```python
from build123d import *

# Parameters (mm, degrees)
BOSS_EXTRUDE1_DEPTH        = 5
BOSS_EXTRUDE1_DEPTH_BACK   = 5
BOSS_EXTRUDE1_2_DEPTH      = 5
BOSS_EXTRUDE1_2_DEPTH_BACK = 5
BOSS_EXTRUDE1_3_DEPTH      = 5
BOSS_EXTRUDE1_3_DEPTH_BACK = 5
BOSS_EXTRUDE2_DEPTH        = 10
BOSS_EXTRUDE2_DEPTH_BACK   = 10
SKETCH1_6_R                = 40
SKETCH1_6_R_2              = 25


with BuildPart() as part:
    # Sketch1 → Boss-Extrude1 (new, two sides: drawn at the far end of the back side and taken through both)
    with BuildSketch(Plane.XY.offset(-BOSS_EXTRUDE1_DEPTH_BACK)):
        with BuildLine():
            Line((10, 47.870166538), (10, -47.870166538))
            ThreePointArc((10, -47.870166538), (0, -46.6), (-10, -47.870166538))
            Line((-10, -47.870166538), (-10, 47.870166538))
            ThreePointArc((-10, 47.870166538), (0, 46.6), (10, 47.870166538))
        make_face()
    extrude(amount=BOSS_EXTRUDE1_DEPTH + BOSS_EXTRUDE1_DEPTH_BACK)



with BuildPart() as body_2:
    # Sketch1 → Boss-Extrude1 2 (new, two sides: drawn at the far end of the back side and taken through both)
    with BuildSketch(Plane.XY.offset(-BOSS_EXTRUDE1_2_DEPTH_BACK)):
        with BuildLine():
            Line((-122.049730922, 28.614375032), (-38.604515092, 76.126633087))
            ThreePointArc((-38.604515092, 76.126633087), (-34.719424314, 66.736425918), (-28.593413405, 58.628287327))
            Line((-28.593413405, 58.628287327), (-111.528626884, 10.952326263))
            ThreePointArc((-111.528626884, 10.952326263), (-115.635110511, 20.470817531), (-122.049730922, 28.614375032))
        make_face()
    extrude(amount=BOSS_EXTRUDE1_2_DEPTH + BOSS_EXTRUDE1_2_DEPTH_BACK)


with BuildPart() as body_3:
    # Sketch1 → Boss-Extrude1 3 (new, two sides: drawn at the far end of the back side and taken through both)
    with BuildSketch(Plane.XY.offset(-BOSS_EXTRUDE1_3_DEPTH_BACK)):
        with BuildLine():
            Line((-111.528626884, -10.952326263), (-28.593413405, -58.628287327))
            ThreePointArc((-28.593413405, -58.628287327), (-34.719424235, -66.736425963), (-38.604515092, -76.126633087))
            Line((-38.604515092, -76.126633087), (-122.049730922, -28.614375032))
            ThreePointArc((-122.049730922, -28.614375032), (-115.635110511, -20.470817531), (-111.528626884, -10.952326263))
        make_face()
    extrude(amount=BOSS_EXTRUDE1_3_DEPTH + BOSS_EXTRUDE1_3_DEPTH_BACK)


with BuildPart() as part_1:
    add(part.part)

    add(body_2.part)  # Boss-Extrude2 merges body 2

    add(body_3.part)  # Boss-Extrude2 merges body 3
    # Sketch1<6> → Boss-Extrude2 (add, two sides: drawn at the far end of the back side and taken through both)
    # profile 1 of 3: a face of its own
    with BuildSketch(Plane.XY.offset(-BOSS_EXTRUDE2_DEPTH_BACK)):
        with Locations((0, 86.6)):
            Circle(SKETCH1_6_R)
        with Locations((0, 86.6)):
            Circle(SKETCH1_6_R_2, mode=Mode.SUBTRACT)
    # profile 2 of 3: a face of its own
    with BuildSketch(Plane.XY.offset(-BOSS_EXTRUDE2_DEPTH_BACK)):
        with Locations((0, -86.6)):
            Circle(SKETCH1_6_R)
        with Locations((0, -86.6)):
            Circle(SKETCH1_6_R_2, mode=Mode.SUBTRACT)
    # profile 3 of 3: a face of its own
    with BuildSketch(Plane.XY.offset(-BOSS_EXTRUDE2_DEPTH_BACK)):
        with Locations((-150, 0)):
            Circle(SKETCH1_6_R)
        with Locations((-150, 0)):
            Circle(SKETCH1_6_R_2, mode=Mode.SUBTRACT)
    extrude(amount=BOSS_EXTRUDE2_DEPTH + BOSS_EXTRUDE2_DEPTH_BACK)


solid = part_1.part
```
Model file for the job. Use its own axes, mm. A direction names the side the tool comes from. Give positions to 0.01 mm unless a question says otherwise; leave off trailing zeros. Write each loop counter-clockwise with the first axis right and the second up, starting at its lowest first coordinate (ties: lowest second). Pieces come first, ordered by that corner, then holes. Notation, with made-up numbers: (67, 30) - (103, 30) arc R18 cw to (103, 61) - close; hole circle Ø6 at (19, -32). An arc over 180 degrees is marked (long way). One line per question, with ' | ' between items. Start each with the question number.
(1) Pin check, flat tips, straight feed: P1, Ø12, axis at x = -112, z = 2, coming from the -Y side; P2, Ø1.5, axis at y = -76, z = 2.5, coming from the -X side; P3, Ø5, axis at y = 2, z = -2.5, coming from the +X side. Stop position of each tip, or through.
(2) Wall check: line 1 along Y through (x, z) = (0, -0.5); line 2 along Y through (x, z) = (-151, -9); line 3 along X through (y, z) = (6, -3.25). Give the ranges that are in metal, low to high. Write a range as from..to.
(3) Slice it at D-D on y = 0. Write the cut outline in (x, z).
(4) Slice it at C-C on z = 0.5. Write the cut outline in (x, y).
(5) 3-axis set-ups, long thin cutter, end or side, ignore diameter. For faces 1 (the face through (-10, -1, 0)), 2 (the face through (10, 1, 0)), 3 (the face through (17, -68, -10)): which of +Z, -Z, +X, -X, +Y, -Y reach the whole face in a straight line?
(6) Slice it at A-A on x = -150. Write the cut outline in (y, z), plus the area to 3 significant figures.
(7) Two-plate mould, pull along Y, no slides. Class faces 4 (the face through (17.22, 104.94, 10)), 5 (the face through (21.5, 120.33, -0.14)): +Y half, -Y half, draft (parallel to the pull), parting line (faces both ways), or undercut.
Results below:
1) P1: y = -37.75 | P2: x = -40.14 | P3: x = 10
2) line 1: -126.6..-111.6, -61.6..61.6, 111.6..126.6 | line 2: -39.99..-24.98, 24.98..39.99 | line 3: -189.55..-174.27, -125.73..-110.45, -10..10
3) outline: (-190, -10) - (-175, -10) - (-175, 10) - (-190, 10) - close; (-125, -10) - (-110, -10) - (-110, 10) - (-125, 10) - close; (-10, -5) - (10, -5) - (10, 5) - (-10, 5) - close
4) outline: (-122.05, -28.61) - (-38.6, -76.13) arc R40 ccw (long way) to (10, -47.87) - (10, 47.87) arc R40 ccw (long way) to (-38.6, 76.13) - (-122.05, 28.61) arc R40 ccw (long way) to start; hole circle Ø50 at (-150, 0); hole (-111.53, -10.95) - (-28.59, -58.63) arc R40 cw to (-10, -47.87) - (-10, 47.87) arc R40 cw to (-28.59, 58.63) - (-111.53, 10.95) arc R40 cw to start; hole circle Ø50 at (0, -86.6); hole circle Ø50 at (0, 86.6)
5) face 1: +Z, -Z | face 2: +Z, -Z, +X | face 3: -Z, +X, -X, +Y, -Y
6) outline: (-40, -10) - (-25, -10) - (-25, 10) - (-40, 10) - close; (25, -10) - (40, -10) - (40, 10) - (25, 10) - close | area: 600 mm^2
7) face 4: draft | face 5: undercut
